from build123d import *

# Parameters (mm, degrees)
SKETCH_1_W                 = 9
SKETCH_1_H                 = 7
EXTRUDE_1_DEPTH            = 180
CUT_EXTRUDE_1_DEPTH        = 1
CUT_EXTRUDE_1_DEPTH_BACK   = 8
CHAMFER_1_SIZE             = 2
CHAMFER_1_SIZE2            = 1.154700538
HOLE_WIZARD_M31_AT_2_COUNT = 2
HOLE_WIZARD_M31_AT_2_PITCH = 50
HOLE_WIZARD_M31_AT_3_COUNT = 2
HOLE_WIZARD_M31_AT_3_PITCH = 100
HOLE_WIZARD_M31_AT_4_COUNT = 2
HOLE_WIZARD_M31_AT_4_PITCH = 150
HOLE_WIZARD_M32_AT_2_COUNT = 2
HOLE_WIZARD_M32_AT_2_PITCH = 50
HOLE_WIZARD_M32_AT_3_COUNT = 2
HOLE_WIZARD_M32_AT_3_PITCH = 110
HOLE_WIZARD_M32_AT_4_COUNT = 2
HOLE_WIZARD_M32_AT_4_PITCH = 160


with BuildPart() as part:
    # Эскиз1 → Бобышка-Вытянуть1 (new body)
    with BuildSketch(Plane.XY):
        with Locations((4.5, 3.5)):
            Rectangle(SKETCH_1_W, SKETCH_1_H)
    extrude(amount=EXTRUDE_1_DEPTH)

    # Эскиз6 → Вырез-Вытянуть1 (cut, two sides)
    with BuildSketch(Plane.XZ) as cut_extrude_1_sk:
        with BuildLine():
            Line((-44.220662013, -367.363162821), (2.062746067, 0))
            ThreePointArc((2.062746067, 0), (4.343145751, 4.656854249), (9, 6.937253933))
            Line((9, 6.937253933), (376.363162821, 53.220662013))
            Line((376.363162821, 53.220662013), (900.000150172, -470.416325339))
            Line((900.000150172, -470.416325339), (479.416325339, -891.000150172))
            Line((479.416325339, -891.000150172), (-44.220662013, -367.363162821))
        make_face()
    extrude(amount=CUT_EXTRUDE_1_DEPTH, mode=Mode.SUBTRACT)
    extrude(cut_extrude_1_sk.sketch, amount=-CUT_EXTRUDE_1_DEPTH_BACK, mode=Mode.SUBTRACT)

    # Фаска1
    chamfer_1_edges = [part.edges().sort_by_distance(p)[0] for p in [
        (9, 7, 93.468626967),
    ]]
    chamfer_1_side = [part.faces().sort_by_distance(p)[0] for p in [
        (9, 3.5, 93.468626967),
    ]]
    chamfer(chamfer_1_edges, length=CHAMFER_1_SIZE, length2=CHAMFER_1_SIZE2, reference=chamfer_1_side[0])

    # Эскиз2 → Отверстие обработанное метчиком M31 (revolve, cut)
    with BuildSketch(Plane(origin=(5, 0, 15), x_dir=(0, 0, -1), z_dir=(1, 0, 0))):
        Polygon((0, 0), (0, 7), (1.75, 7), (1.25, 6.5), (1.25, 0.5), (1.75, 0), align=None)
    hole_wizard_m31 = revolve(axis=Axis((5, -6.35, 15), (0, 1, 0)), mode=Mode.SUBTRACT)

    # Отверстие обработанное метчиком M31 at 2: Отверстие обработанное метчиком M31 ×2
    with Locations(*[(0, 0, i * HOLE_WIZARD_M31_AT_2_PITCH) for i in range(1, HOLE_WIZARD_M31_AT_2_COUNT)]):
        add(hole_wizard_m31, mode=Mode.SUBTRACT)

    # Отверстие обработанное метчиком M31 at 3: Отверстие обработанное метчиком M31 ×2
    with Locations(*[(0, 0, i * HOLE_WIZARD_M31_AT_3_PITCH) for i in range(1, HOLE_WIZARD_M31_AT_3_COUNT)]):
        add(hole_wizard_m31, mode=Mode.SUBTRACT)

    # Отверстие обработанное метчиком M31 at 4: Отверстие обработанное метчиком M31 ×2
    with Locations(*[(0, 0, i * HOLE_WIZARD_M31_AT_4_PITCH) for i in range(1, HOLE_WIZARD_M31_AT_4_COUNT)]):
        add(hole_wizard_m31, mode=Mode.SUBTRACT)

    # Эскиз4 → Отверстие обработанное метчиком M32 (revolve, cut)
    with BuildSketch(Plane(origin=(0, 4, 10), x_dir=(0, 0, 1), z_dir=(0, 1, 0))):
        Polygon((0, 0), (0, 9), (1.75, 9), (1.25, 8.5), (1.25, 0.5), (1.75, 0), align=None)
    hole_wizard_m32 = revolve(axis=Axis((-6.35, 4, 10), (1, 0, 0)), mode=Mode.SUBTRACT)

    # Отверстие обработанное метчиком M32 at 2: Отверстие обработанное метчиком M32 ×2
    with Locations(*[(0, 0, i * HOLE_WIZARD_M32_AT_2_PITCH) for i in range(1, HOLE_WIZARD_M32_AT_2_COUNT)]):
        add(hole_wizard_m32, mode=Mode.SUBTRACT)

    # Отверстие обработанное метчиком M32 at 3: Отверстие обработанное метчиком M32 ×2
    with Locations(*[(0, 0, i * HOLE_WIZARD_M32_AT_3_PITCH) for i in range(1, HOLE_WIZARD_M32_AT_3_COUNT)]):
        add(hole_wizard_m32, mode=Mode.SUBTRACT)

    # Отверстие обработанное метчиком M32 at 4: Отверстие обработанное метчиком M32 ×2
    with Locations(*[(0, 0, i * HOLE_WIZARD_M32_AT_4_PITCH) for i in range(1, HOLE_WIZARD_M32_AT_4_COUNT)]):
        add(hole_wizard_m32, mode=Mode.SUBTRACT)


solid = part.part
Work out the finished part from the listing and answer in its coordinate system (mm). Round coordinates to 2 decimals unless told otherwise and drop trailing zeros. Write each loop counter-clockwise with the first axis right and the second up, starting at its lowest first coordinate (ties: lowest second). Pieces come first, ordered by that corner, then holes.
1) Given pin 1 Ø3 at (x, z) = (5, 65) entering from +Y; pin 2 Ø1 at (x, y) = (6, 1.5) entering from -Z, each flat-ended and moving along its own axis, determine where each tip first touches the part or whether it passes through.
2) Straight lines are drawn through the part: line 1 (Y direction, x = 5.75, z = 10); line 2 (X direction, y = 5.05, z = 65); line 3 (Z direction, x = 7.75, y = 4.5). For each, find the intervals that lie inside material, in ascending order.
3) The mould has two halves that part along X. Classify faces 1 (the flat face through (9, 2, 92)), 2 (the flat face through (4, 0, 89)): pulls with the +X half, pulls with the -X half, needs draft (parallel to the pull), parting line crosses it, or undercut.
4) A cutting plane is placed at A-A (z = 161.5). Give the vertices of the cut face in (x, y).
Completed:
1. pin 1: stops at y = 6.75
1. pin 2: stops at z = 5.61
2. line 1: y = 0 to 2.75, 5.25 to 7
2. line 2: x = 0 to 3.75, 6.25 to 8.97
2. line 3: z = 6.68 to 8.85, 11.15 to 58.85, 61.15 to 118.85, 121.15 to 168.85, 171.15 to 180
3. face 1: pulls with the +X half
3. face 2: needs draft
4. outline: (0, 0) - (9, 0) - (9, 5) - (7.85, 7) - (0, 7) - close
